Part print with two shaded views. Sizes in mm from the minimum x, y, z corner. Round coordinates to 2 decimals unless told otherwise and drop trailing zeros. Order: outer loops, then holes, each group sorted by start corner. A loop starts at its lowest first (then second) coordinate and runs counter-clockwise, first axis right, second up. Notation, with made-up numbers: (-23, -0.5) -> (-9, -0.5) arc R16 ccw to (-9, 19.5) -> close; hole circle Ø10 at (-5, 47.25). An arc over 180 degrees is marked (long way). Answer as a JSON object with one key per item and string values.
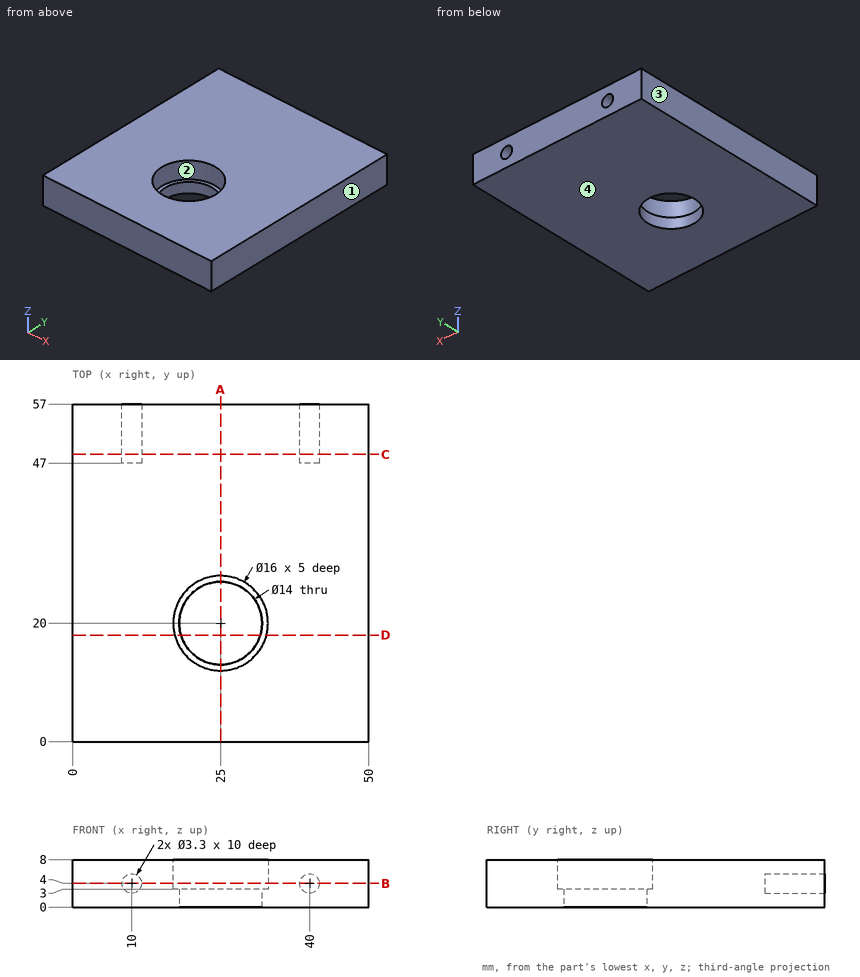
1) Probe L1, parallel to X at y = 54.5, z = 4; L2, parallel to Y at x = 25, z = 5.2; L3, parallel to Y at x = 25, z = 2.25. List the from-to ranges inside material, lowest first. Write a range as from..to.
Checked values:
{"L1": "x = 0..8.35, 11.65..38.35, 41.65..50", "L2": "y = 0..12, 28..57", "L3": "y = 0..13, 27..57"}
2) Flat gauge pin, fed straight in: pin 1 Ø1.6 at (x, z) = (9.5, 3.5) entering from +Y. Where does the tip first touch, or does it go through?
Checked values:
{"pin 1": "stops at y = 47"}
3) Cut at C-C, the plane y = 48.5. Give the cut face in (x, z).
Checked values:
{"outline": "(0, 0) -> (50, 0) -> (50, 8) -> (0, 8) -> close; hole circle Ø3.3 at (10, 4); hole circle Ø3.3 at (40, 4)"}
4) Cut at D-D, the plane y = 18. Give the cut face in (x, z), plus the area to 3 significant figures.
Checked values:
{"outline": "(0, 0) -> (18.29, 0) -> (18.29, 3) -> (17.25, 3) -> (17.25, 8) -> (0, 8) -> close; (31.71, 0) -> (50, 0) -> (50, 8) -> (32.75, 8) -> (32.75, 3) -> (31.71, 3) -> close", "area": "282 mm²"}
5) Cut at B-B, the plane z = 4. Give the cut face in (x, y), plus the area to 3 significant figures.
Checked values:
{"outline": "(0, 0) -> (50, 0) -> (50, 57) -> (41.65, 57) -> (41.65, 47) -> (38.35, 47) -> (38.35, 57) -> (11.65, 57) -> (11.65, 47) -> (8.35, 47) -> (8.35, 57) -> (0, 57) -> close; hole circle Ø16 at (25, 20)", "area": "2,580 mm²"}
6) Pull direction X, two halves, no side cores. Call the marked faces 1, 2, 3 and 4: pulls with the +X half, pulls with the -X half, needs draft (parallel to the pull), parting line crosses it, or undercut.
Checked values:
{"face 1": "pulls with the +X half", "face 2": "undercut", "face 3": "pulls with the -X half", "face 4": "needs draft"}
7) Cut at A-A, the plane x = 25. Give the cut face in (y, z), plus the area to 3 significant figures.
Checked values:
{"outline": "(0, 0) -> (13, 0) -> (13, 3) -> (12, 3) -> (12, 8) -> (0, 8) -> close; (27, 0) -> (57, 0) -> (57, 8) -> (28, 8) -> (28, 3) -> (27, 3) -> close", "area": "334 mm²"}
